Can you work these out from the model? Positions are in its coordinate system, mm. Face numbers are marked on the shaded views. A direction names the side the tool comes from. Coordinates: 2 decimals unless noted, no trailing zeros. Order: outer loops, then holes, each group sorted by start corner. A loop starts at its lowest first (then second) coordinate and runs counter-clockwise, first axis right, second up. Notation, with made-up numbers: (62, 35.5) -> (86, 35.5) arc R12 ccw to (86, 44.5) -> close; hole circle Ø5 at (-10.75, 60). An arc over 180 degrees is marked (long way). Answer as CSV lines item,"result".
from build123d import *

# Parameters (mm, degrees)
F1_DEPTH = 25.4


with BuildPart() as f1:
    # F0 (on Front) → F1 (new body)
    with BuildSketch(Plane.XZ):
        with BuildLine():
            Line((-29.147431, 26.136464), (-39.287967, 26.136464))
            ThreePointArc((-39.287967, 26.136464), (-41.136623, 17.396081), (-33.380877, 12.962096))
            Line((-33.380877, 12.962096), (-20.243494, 12.962096))
            Line((-20.243494, 12.962096), (-19.404731, 20.111647))
            Line((-19.404731, 20.111647), (-18.697919, 26.136464))
            Line((-18.697919, 26.136464), (-28.992943, 26.136464))
            Line((-28.992943, 26.136464), (-29.147431, 26.136464))
        make_face()
    extrude(amount=F1_DEPTH)


solid = f1.part
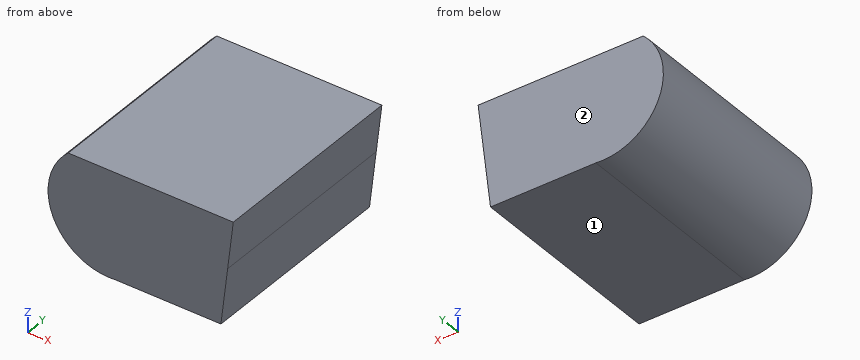
Q1. If I drill on line 1 (Z direction, x = -33.25, y = -9.25); line 2 (X direction, y = -22.75, z = 19); line 3 (Z direction, x = -35.75, y = -23.75), over which ranges is the centre line in solid material (lowest first)?
Solution:
line 1,"12.96 to 26.14"
line 2,"-41.65 to -19.54"
line 3,"13.07 to 26.14"
Q2. Imagine slicing it at B-B (x = -36.25). List the corners of the cut face in (y, z) for me.
Solution:
outline,"(-25.4, 13.19) -> (0, 13.19) -> (0, 26.14) -> (-25.4, 26.14) -> close"
Q3. Imagine slicing it at C-C (z = 19.5). List the corners of the cut face in (x, y) for me.
Solution:
outline,"(-41.73, -25.4) -> (-19.48, -25.4) -> (-19.48, 0) -> (-41.73, 0) -> close"
Q4. Which directions (+Z, -Z, +X, -X, +Y, -Y) give clear straight access to the entire face, cutting with the end or side of a thin tool? Please do the marked faces 1 and 2.
Solution:
face 1,"-Z, +X, +Y, -Y"
face 2,"+Z, -Z, +X, -X, +Y"
Q5. Imagine slicing it at A-A (y = -19.75). List the corners of the cut face in (x, z) for me, and give its area (3 significant figures).
Solution:
outline,"(-39.29, 26.14) arc R7.58 ccw to (-33.38, 12.96) -> (-20.24, 12.96) -> (-19.4, 20.11) -> (-18.7, 26.14) -> close"
area,"278 mm2"
Q6. For P1, Ø1, axis at x = -32.5, y = -20.5, coming from the -Z side; P2, Ø4, axis at y = -7.5, z = 15, coming from the +X side, each with a flat end and sliding along its axis, tell me the tip position at first contact or that it passes through.
Solution:
P1,"z = 12.96"
P2,"x = -19.77"
